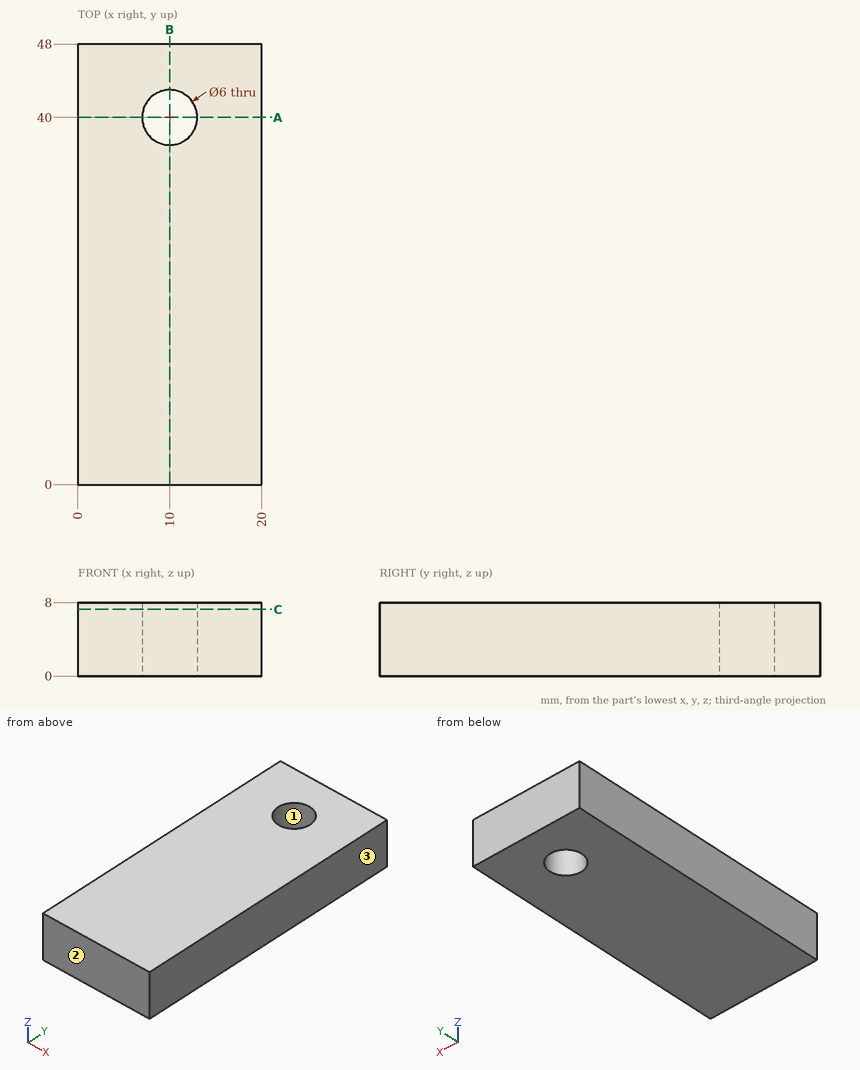
The figure shows three views and two pictorial views of one solid part (mm, origin at its lowest corner). Answer the questions. Coordinates: 2 decimals unless noted, no trailing zeros. Loops run counter-clockwise (first coordinate to the right, second up) from the corner with the lowest first, then second, coordinate; pieces in that order, holes last. Notation, with made-up numbers: (40.25, 29.5) - (47.25, 29.5) arc R35 ccw to (47.25, 64.5) - close; hole circle Ø11 at (-40, -36.75). An arc over 180 degrees is marked (long way). Use a Markdown table: item, result. Add a question column.
1) Find the intervals of material crossed by line 1 (Y direction, x = 10, z = 4.25); line 2 (X direction, y = 40, z = 5.25); line 3 (Y direction, x = 12.5, z = 6), in increasing order.
2) The part is cut by section A-A, the plane y = 40. Give the vertices of the cut face in (x, z).
3) The mould has two halves that part along X. Classify the marked faces 1, 2 and 3: released by +X, released by -X, zero draft, split by the parting line, or undercut.
4) The part is cut by section C-C, the plane z = 7.25. Give the vertices of the cut face in (x, y), and give its area (3 significant figures).
5) The part is cut by section B-B, the plane x = 10. Give the vertices of the cut face in (y, z).
Here are the results:
| question | item | result |
|---|---|---|
| 1 | line 1 | y = 0 to 37, 43 to 48 |
| 1 | line 2 | x = 0 to 7, 13 to 20 |
| 1 | line 3 | y = 0 to 38.34, 41.66 to 48 |
| 2 | outline | (0, 0) - (7, 0) - (7, 8) - (0, 8) - close; (13, 0) - (20, 0) - (20, 8) - (13, 8) - close |
| 3 | face 1 | undercut |
| 3 | face 2 | zero draft |
| 3 | face 3 | released by +X |
| 4 | outline | (0, 0) - (20, 0) - (20, 48) - (0, 48) - close; hole circle Ø6 at (10, 40) |
| 4 | area | 932 mm^2 |
| 5 | outline | (0, 0) - (37, 0) - (37, 8) - (0, 8) - close; (43, 0) - (48, 0) - (48, 8) - (43, 8) - close |
